Model file for the job. Use its own axes, mm. A direction names the side the tool comes from. Coordinates: 2 decimals unless noted, no trailing zeros. Write each loop counter-clockwise with the first axis right and the second up, starting at its lowest first coordinate (ties: lowest second). Pieces come first, ordered by that corner, then holes.
Q1. Band-saw the part on D-D, the plane z = 69. Write the cut outline in (x, y).
Q2. Band-saw the part on C-C, the plane x = -32.5. Write the cut outline in (y, z).
Q3. Which spindle directions (+Z, -Z, +X, -X, +Y, -Y) get a long thin tool onto all of the face, cutting with end or side? Do faces 4 (the flat face through (-48, 4, 107.95)), 5 (the flat face through (6.35, 4, 75)), 6 (the cylindrical face through (6.19, 6.37, 2.82)), 7 (the flat face through (-8, 7.62, 81)). Say none if no direction does.
Q4. Pull direction X, two halves, no side cores. Call faces 1 (the flat face through (10, 5.08, 14)), 2 (the cylindrical face through (-40.34, 3.76, 107.45)), 3 (the cylindrical face through (20.242, 3.863, 118.854)): released by +X, released by -X, zero draft, split by the parting line, or undercut.
Q5. Band-saw the part on B-B, the plane z = 16.51. Write the cut outline in (x, y) (3 decimals).
Q6. Drill centre lines: probe 1 along Z at (x, y) = (8.89, 2); probe 2 along X at (y, z) = (1.1, 6.35); probe 3 along X at (y, z) = (6.6, 6.35) (3 decimals). Where is each one in solid material? Low to high.
Q7. Band-saw the part on A-A, the plane y = 2. State how many separate pieces and enclosed holes the cut face has, plus the area to 3 significant figures.
Q8. Pin check, flat tips, straight feed: P1, Ø2.5, axis at y = 2, z = 15, coming from the +X side; P2, Ø2.5, axis at y = 3, z = 13, coming from the -X side; P3, Ø10, axis at x = 7.5, z = 15, coming from the +Y side; P4, Ø2.5, axis at y = 4.5, z = 63.5, coming from the -X side. Stop position of each tip, or through.
from build123d import *

# Parameters (mm, degrees)
SKETCH1_R           = 2.286
BOSS_EXTRUDE1_DEPTH = 7.62
FILLET1_R           = 25.4
FILLET3_R           = 44.45
FILLET2_R           = 6.35
FILLET4_R           = 31.75
SKETCH3_R           = 4.445
CUT_EXTRUDE1_DEPTH  = 2.54
FILLET5_R           = 2.54


# Some blends are built 0.0001 mm under size
with BuildPart() as part:
    # Sketch1 → Boss-Extrude1 (new body)
    with BuildSketch(Plane(origin=(0, 0, 0), x_dir=(1, 0, 0), z_dir=(0, 1, 0))):
        Polygon((0, 0), (17.78, 0), (17.78, -25.4), (6.35, -50.8), (6.35, -107.95), (26.67, -120.65), (-55.88, -120.65), (-55.88, -107.95), (-5.08, -107.95), (-11.43, -90.17), (-11.43, -50.8), (0, -25.4), align=None)
        with Locations(Location((8.89, -6.35, 0), (0, 0, 270))):
            Circle(SKETCH1_R, mode=Mode.SUBTRACT)
        with Locations(Location((8.89, -16.51, 0), (0, 0, 270))):
            Circle(SKETCH1_R, mode=Mode.SUBTRACT)
    extrude(amount=BOSS_EXTRUDE1_DEPTH)

    # Fillet1
    fillet1_edges = [part.edges().sort_by_distance(p)[0] for p in [
        (17.78, 3.81, 25.4),
        (6.35, 3.81, 50.8),
        (6.35, 3.81, 107.95),
        (-11.43, 3.81, 50.8),
        (0, 3.81, 25.4),
    ]]
    fillet(fillet1_edges, radius=FILLET1_R)

    # Fillet3
    # the kernel refuses this fillet: 44.45 mm, written as the material it adds along each edge
    with BuildSketch(Plane(origin=(-5.08, 0, 107.95), x_dir=(-0.3363363969981565, 0, -0.9417419115948374), z_dir=(0, 1, 0))) as fillet3_piece_1:
        with BuildLine():
            CenterArc((55.956286369, 24.518250668), FILLET3_R, 160.346175942, 53.130102354)
            Line((14.095858398, 39.468403515), (13.258649839, 39.767406572))
            Line((13.258649839, 39.767406572), (-0.837208559, 0.299003057))
            Line((-0.837208559, 0.299003057), (0, -0.889))
            ThreePointArc((0, -0.889), (9.439953655, -0.889), (18.138379728, -0.490365013))
            Line((18.138379728, -0.490365013), (18.879907309, 0))
        make_face()
    extrude(amount=7.62)

    # Fillet2
    fillet2_edges = [part.edges().sort_by_distance(p)[0] for p in [
        (17.78, 3.81, 0),
        (0, 3.81, 0),
        (-55.88, 3.81, 120.65),
        (-55.88, 3.81, 107.95),
    ]]
    fillet(fillet2_edges, radius=FILLET2_R - 0.0001)  # a hair under: the kernel refuses the full size

    # Fillet4
    fillet4_edges = [part.edges().sort_by_distance(p)[0] for p in [
        (-11.43, 3.81, 90.17),
    ]]
    fillet(fillet4_edges, radius=FILLET4_R)

    # Sketch3 → Cut-Extrude1 (cut)
    with BuildSketch(Plane(origin=(0, 7.62, 0), x_dir=(1, 0, 0), z_dir=(0, 1, 0))):
        with Locations(Location((8.89, -6.35, 0), (0, 0, 270))):
            Circle(SKETCH3_R)
        with Locations(Location((8.89, -16.51, 0), (0, 0, 270))):
            Circle(SKETCH3_R)
    extrude(amount=-CUT_EXTRUDE1_DEPTH, mode=Mode.SUBTRACT)

    # Fillet5
    fillet5_edges = [part.edges().sort_by_distance(p)[0] for p in [
        (26.67, 3.81, 120.65),
    ]]
    fillet(fillet5_edges, radius=FILLET5_R)


solid = part.part
Answer sheet:
1. outline: (-11.43, 0) - (6.35, 0) - (6.35, 7.62) - (-11.43, 7.62) - close
2. outline: (0, 105.51) - (7.62, 105.51) - (7.62, 120.65) - (0, 120.65) - close
3. face 4: -Z, -X, +Y, -Y
3. face 5: +X, +Y, -Y
3. face 6: +Y
3. face 7: +Z, -Z, +X, -X, +Y
4. face 1: undercut
4. face 2: released by -X
4. face 3: released by +X
5. outline: (0, 0) - (6.604, 0) - (6.604, 5.08) - (4.445, 5.08) - (4.445, 7.62) - (0, 7.62) - close; (11.176, 0) - (17.78, 0) - (17.78, 7.62) - (13.335, 7.62) - (13.335, 5.08) - (11.176, 5.08) - close
6. probe 1: z = 0 to 4.06, 8.64 to 14.22, 18.8 to 45.16, 104.94 to 120.65
6. probe 2: x = 0 to 6.6, 11.18 to 17.78
6. probe 3: x = 0 to 4.445, 13.335 to 17.78
7. separate pieces: 1
7. enclosed holes: 2
7. area: 3,020 mm2
8. P1: stops at x = 17.78
8. P2: stops at x = 0
8. P3: stops at y = 7.62
8. P4: stops at x = -11.43
